For this review, take the finished solid that the model builds, in its own axes (mm). A direction names the side the tool comes from. Give positions to 0.01 mm unless a question says otherwise; leave off trailing zeros. Write each loop counter-clockwise with the first axis right and the second up, starting at its lowest first coordinate (ties: lowest second). Pieces come first, ordered by that corner, then holes. Notation, with made-up numbers: (6, -11.75) -> (21, -11.75) arc R25 ccw to (21, 25.25) -> close; hole circle Ø1 at (-38, 69). An arc over 180 degrees is marked (long way). Return JSON: item names as keys, results as strings.
from build123d import *

# Parameters (mm, degrees)
SKETCH_W      = 180
SKETCH_H      = 180
SKETCH_R      = 2
PAD_DEPTH     = 5
SKETCH001_R   = 4
SKETCH001_R_2 = 2
PAD001_DEPTH  = 3


with BuildPart() as part:
    # Sketch → Pad (new body)
    with BuildSketch(Plane.XY):
        with Locations((90, 90)):
            Rectangle(SKETCH_W, SKETCH_H)
        with Locations((15, 30)):
            Circle(SKETCH_R, mode=Mode.SUBTRACT)
        with Locations((15, 81)):
            Circle(SKETCH_R, mode=Mode.SUBTRACT)
        with Locations((60, 30)):
            Circle(SKETCH_R, mode=Mode.SUBTRACT)
        with Locations((60, 81)):
            Circle(SKETCH_R, mode=Mode.SUBTRACT)
        with Locations((120, 150)):
            Circle(SKETCH_R, mode=Mode.SUBTRACT)
        with Locations((165, 150)):
            Circle(SKETCH_R, mode=Mode.SUBTRACT)
        with Locations((120, 99)):
            Circle(SKETCH_R, mode=Mode.SUBTRACT)
        with Locations((165, 99)):
            Circle(SKETCH_R, mode=Mode.SUBTRACT)
        with Locations((10, 16.4)):
            Circle(SKETCH_R, mode=Mode.SUBTRACT)
        with Locations((16.4, 10)):
            Circle(SKETCH_R, mode=Mode.SUBTRACT)
        with Locations((170, 16.4)):
            Circle(SKETCH_R, mode=Mode.SUBTRACT)
        with Locations((163.6, 10)):
            Circle(SKETCH_R, mode=Mode.SUBTRACT)
        with Locations((10, 163.6)):
            Circle(SKETCH_R, mode=Mode.SUBTRACT)
        with Locations((16.4, 170)):
            Circle(SKETCH_R, mode=Mode.SUBTRACT)
        with Locations((163.6, 170)):
            Circle(SKETCH_R, mode=Mode.SUBTRACT)
        with Locations((170, 163.6)):
            Circle(SKETCH_R, mode=Mode.SUBTRACT)
        with Locations((72.1, 155)):
            Circle(SKETCH_R, mode=Mode.SUBTRACT)
        with Locations((20, 149.9)):
            Circle(SKETCH_R, mode=Mode.SUBTRACT)
        with Locations((20, 122)):
            Circle(SKETCH_R, mode=Mode.SUBTRACT)
        with Locations((70.8, 106.8)):
            Circle(SKETCH_R, mode=Mode.SUBTRACT)
        with Locations((107.9, 30)):
            Circle(SKETCH_R, mode=Mode.SUBTRACT)
        with Locations((109.2, 78.2)):
            Circle(SKETCH_R, mode=Mode.SUBTRACT)
        with Locations((160, 63)):
            Circle(SKETCH_R, mode=Mode.SUBTRACT)
        with Locations((160, 35.1)):
            Circle(SKETCH_R, mode=Mode.SUBTRACT)
        with Locations((90, 170)):
            Circle(SKETCH_R, mode=Mode.SUBTRACT)
        with Locations((40, 10)):
            Circle(SKETCH_R, mode=Mode.SUBTRACT)
        with Locations((140, 10)):
            Circle(SKETCH_R, mode=Mode.SUBTRACT)
    extrude(amount=PAD_DEPTH)

    # Sketch001 (on Face33 of Pad) → Pad001 (join)
    with BuildSketch(Plane.XY.offset(5)):
        with Locations((20, 149.9)):
            Circle(SKETCH001_R)
        with Locations((20, 149.9)):
            Circle(SKETCH001_R_2, mode=Mode.SUBTRACT)
        with Locations((72.1, 155)):
            Circle(SKETCH001_R)
        with Locations((72.1, 155)):
            Circle(SKETCH001_R_2, mode=Mode.SUBTRACT)
        with Locations((20, 122)):
            Circle(SKETCH001_R)
        with Locations((20, 122)):
            Circle(SKETCH001_R_2, mode=Mode.SUBTRACT)
        with Locations((70.8, 106.8)):
            Circle(SKETCH001_R)
        with Locations((70.8, 106.8)):
            Circle(SKETCH001_R_2, mode=Mode.SUBTRACT)
        with Locations((15, 81)):
            Circle(SKETCH001_R)
        with Locations((15, 81)):
            Circle(SKETCH001_R_2, mode=Mode.SUBTRACT)
        with Locations((60, 81)):
            Circle(SKETCH001_R)
        with Locations((60, 81)):
            Circle(SKETCH001_R_2, mode=Mode.SUBTRACT)
        with Locations((60, 30)):
            Circle(SKETCH001_R)
        with Locations((60, 30)):
            Circle(SKETCH001_R_2, mode=Mode.SUBTRACT)
        with Locations((15, 30)):
            Circle(SKETCH001_R)
        with Locations((15, 30)):
            Circle(SKETCH001_R_2, mode=Mode.SUBTRACT)
        with Locations((107.9, 30)):
            Circle(SKETCH001_R)
        with Locations((107.9, 30)):
            Circle(SKETCH001_R_2, mode=Mode.SUBTRACT)
        with Locations((160, 35.1)):
            Circle(SKETCH001_R)
        with Locations((160, 35.1)):
            Circle(SKETCH001_R_2, mode=Mode.SUBTRACT)
        with Locations((109.2, 78.2)):
            Circle(SKETCH001_R)
        with Locations((109.2, 78.2)):
            Circle(SKETCH001_R_2, mode=Mode.SUBTRACT)
        with Locations((160, 63)):
            Circle(SKETCH001_R)
        with Locations((160, 63)):
            Circle(SKETCH001_R_2, mode=Mode.SUBTRACT)
        with Locations((120, 99)):
            Circle(SKETCH001_R)
        with Locations((120, 99)):
            Circle(SKETCH001_R_2, mode=Mode.SUBTRACT)
        with Locations((165, 99)):
            Circle(SKETCH001_R)
        with Locations((165, 99)):
            Circle(SKETCH001_R_2, mode=Mode.SUBTRACT)
        with Locations((120, 150)):
            Circle(SKETCH001_R)
        with Locations((120, 150)):
            Circle(SKETCH001_R_2, mode=Mode.SUBTRACT)
        with Locations((165, 150)):
            Circle(SKETCH001_R)
        with Locations((165, 150)):
            Circle(SKETCH001_R_2, mode=Mode.SUBTRACT)
    extrude(amount=PAD001_DEPTH)


solid = part.part
1. To check wall thickness, follow probe 1 along X at (y, z) = (170, 2.2); probe 2 along Y at (x, z) = (20, 3); probe 3 along Y at (x, z) = (119, 6.25). State the ranges of each line that lie inside material, in increasing order.
Results found:
{"probe 1": "x = 0 to 14.4, 18.4 to 88, 92 to 161.6, 165.6 to 180", "probe 2": "y = 0 to 120, 124 to 147.9, 151.9 to 180", "probe 3": "y = 95.13 to 97.27, 100.73 to 102.87, 146.13 to 148.27, 151.73 to 153.87"}
2. For faces 3 (the cylindrical face through (71.723, 105.026, 3.944)), 4 (the cylindrical face through (19.479, 153.866, 6.479)), list the 3-axis set-ups (+Z, -Z, +X, -X, +Y, -Y) from which the entire face can be reached by the end or side of a thin tool; tool diameter is ignored.
Results found:
{"face 3": "+Z, -Z", "face 4": "+Z"}
3. Add section A-A, the plane x = 49.5. State the section outline as (y, z) points, plus the area to 3 significant figures.
Results found:
{"outline": "(0, 0) -> (180, 0) -> (180, 5) -> (0, 5) -> close", "area": "900 mm²"}
4. The part is to be moulded in two halves that separate along Y. For faces 1 (the flat face through (21, 124, 8)), 2 (the cylindrical face through (163.4, 148.8, 3.9)), say which applies: +Y half, -Y half, draft (parallel to the pull), parting line (faces both ways), or undercut.
Results found:
{"face 1": "draft", "face 2": "undercut"}
5. For pin 1 (1.5 mm diameter, centred on y = 65, z = 6, fed in from -X); pin 2 (5 mm diameter, centred on x = 74.5, y = 124, fed in from +Z), all flat-tipped, find the tip position at first contact; note any pin that passes through.
Results found:
{"pin 1": "stops at x = 156.2", "pin 2": "stops at z = 5"}
